from build123d import *

# Parameters (mm, degrees)
SKETCH1_R           = 25.4
SKETCH1_R_2         = 22.225
BOSS_EXTRUDE1_DEPTH = 914.4
CUT_EXTRUDE1_START  = -539.75
SKETCH2_R           = 25.4
CUT_EXTRUDE1_DEPTH  = 376.35528356
CUT_EXTRUDE3_DEPTH  = 541.943973531


with BuildPart() as part:
    # Sketch1 → Boss-Extrude1 (new body)
    with BuildSketch(Plane.XY):
        Circle(SKETCH1_R)
        Circle(SKETCH1_R_2, mode=Mode.SUBTRACT)
    extrude(amount=BOSS_EXTRUDE1_DEPTH)

    # Sketch2 → Cut-Extrude1 (cut, through all)
    with BuildSketch(Plane(origin=(0, 0, 0), x_dir=(-1, 0, 0), z_dir=(0, 0, -1)).offset(CUT_EXTRUDE1_START)):
        Circle(SKETCH2_R)
    extrude(amount=-CUT_EXTRUDE1_DEPTH, mode=Mode.SUBTRACT)

    # Sketch4 → Cut-Extrude3 (cut, through all)
    with BuildSketch(Plane.XY):
        with BuildLine():
            Line((-25.4, 0), (25.4, 0))
            ThreePointArc((25.4, 0), (0, 25.4), (-25.4, 0))
        make_face()
    extrude(amount=CUT_EXTRUDE3_DEPTH, mode=Mode.SUBTRACT)


solid = part.part
Work out the finished part from the listing and answer in its coordinate system (mm). Give positions to 0.01 mm unless a question says otherwise; leave off trailing zeros. Loops run counter-clockwise (first coordinate to the right, second up) from the corner with the lowest first, then second, coordinate; pieces in that order, holes last. Notation, with made-up numbers: (24.25, 19.25) -> (77.25, 19.25) arc R27 ccw to (77.25, 44.25) -> close; hole circle Ø1 at (32.25, 44.25). An arc over 180 degrees is marked (long way). Use a Markdown table: item, result. Add a question column.
1) Each of these flat-tipped pins is pushed along its axis until it touches: P1, Ø8, axis at x = 9.5, z = 335.5, coming from the -Y side; P2, Ø1, axis at x = 14, z = 158.5, coming from the -Y side; P3, Ø2, axis at y = -4.5, z = 205.5, coming from the -X side. Where does it stop, or does it pass through?
2) The part is cut by section C-C, the plane z = 275. Determine the outline of the cut face in (x, y) (3 decimals), plus the area to 3 significant figures.
3) Consider line 1 along X through (y, z) = (-1.5, 311.5); line 2 along X through (y, z) = (-18.5, 87); line 3 along Y through (x, z) = (-1.5, 53.5). Determine where each line is inside the solid, lowest interval first.
4) For a pull along X with two mould halves and no side action, classify faces 1 (the cylindrical face through (-0.559, -25.394, 266.097)), 2 (the flat face through (-4, -23, 0)), 3 (the cylindrical face through (-0.49, -22.22, 266.1)) as +X half, -X half, draft (parallel to the pull), parting line (faces both ways), or undercut.
5) The part is cut by section A-A, the plane y = -14. Determine the outline of the cut face in (x, z), plus the area to 3 significant figures.
6) The part is cut by section B-B, the plane x = 0. Determine the outline of the cut face in (y, z) (3 decimals), plus the area to 3 significant figures.
Reported:
| question | item | result |
|---|---|---|
| 1 | P1 | stops at y = -24.8 |
| 1 | P2 | stops at y = -21.52 |
| 1 | P3 | stops at x = -25.16 |
| 2 | outline | (-25.4, 0) arc R25.4 ccw to (25.4, 0) -> (22.225, 0) arc R22.225 cw to (-22.225, 0) -> close |
| 2 | area | 238 mm^2 |
| 3 | line 1 | x = -25.36 to -22.17, 22.17 to 25.36 |
| 3 | line 2 | x = -17.4 to -12.32, 12.32 to 17.4 |
| 3 | line 3 | y = -25.36 to -22.17 |
| 4 | face 1 | parting line |
| 4 | face 2 | draft |
| 4 | face 3 | undercut |
| 5 | outline | (-21.19, 0) -> (-17.26, 0) -> (-17.26, 539.75) -> (-21.19, 539.75) -> close; (17.26, 0) -> (21.19, 0) -> (21.19, 539.75) -> (17.26, 539.75) -> close |
| 5 | area | 4,240 mm^2 |
| 6 | outline | (-25.4, 0) -> (-22.225, 0) -> (-22.225, 539.75) -> (-25.4, 539.75) -> close |
| 6 | area | 1,710 mm^2 |
